from build123d import *

# Parameters (mm, degrees)
DODANIE_WYCI_GNI_CIE1_DEPTH = 6
SZKIC3_R                    = 21.25
WYTNIJ_WYCI_GNI_CIE1_DEPTH  = 10
SZKIC4_R                    = 1.55
WYTNIJ_WYCI_GNI_CIE2_DEPTH  = 10


with BuildPart() as part:
    # Szkic1 → Dodanie-wyciągnięcie1 (new body)
    with BuildSketch(Plane.XY):
        with BuildLine():
            ThreePointArc((38.780616011, 73.907751151), (41.279513808, -10.21802082), (43.778411605, 73.907751151))
            ThreePointArc((43.778411605, 73.907751151), (41.279513808, 76.48197918), (38.780616011, 73.907751151))
        make_face()
    extrude(amount=DODANIE_WYCI_GNI_CIE1_DEPTH)

    # Szkic3 → Wytnij-wyciągnięcie1 (cut)
    with BuildSketch(Plane.XY.offset(6)):
        with Locations((41.279513808, 21.88197918)):
            Circle(SZKIC3_R)
    extrude(amount=-WYTNIJ_WYCI_GNI_CIE1_DEPTH, mode=Mode.SUBTRACT)

    # Szkic4 → Wytnij-wyciągnięcie2 (cut)
    with BuildSketch(Plane.XY.offset(6)):
        with Locations((41.279513808, -5.11802082)):
            Circle(SZKIC4_R)
        with Locations((17.896827906, 35.38197918)):
            Circle(SZKIC4_R)
        with Locations((64.66219971, 35.38197918)):
            Circle(SZKIC4_R)
        with Locations((41.279513808, 66.88197918)):
            Circle(SZKIC4_R)
    extrude(amount=-WYTNIJ_WYCI_GNI_CIE2_DEPTH, mode=Mode.SUBTRACT)


solid = part.part
For this review, take the finished solid that the model builds, in its own axes (mm). Round coordinates to 2 decimals unless told otherwise and drop trailing zeros. Order: outer loops, then holes, each group sorted by start corner. A loop starts at its lowest first (then second) coordinate and runs counter-clockwise, first axis right, second up. Notation, with made-up numbers: (-17, 31.5) -> (4, 31.5) arc R13 cw to (4, 35.5) -> close; hole circle Ø10 at (49.5, 21.25). An arc over 180 degrees is marked (long way). Write item = value, one per line. Start each with the question number.
1) Insertion check: pin 1 (3 mm diameter, centred on x = 64.66, y = 35.38, fed in from -Z); pin 2 (3 mm diameter, centred on x = 36.5, z = 4.5, fed in from -Y); pin 3 (2 mm diameter, centred on y = 66, z = 4, fed in from +X); pin 4 (2 mm diameter, centred on y = 54.5, z = 1, fed in from -X). Each pin has a flat end and moves straight along its axis. Give the tip position at first contact, or say it passes through.
2) Take a section at A-A on x = 29.5. State the section outline as (y, z) points, plus the area to 3 significant figures.
3) The part is to be moulded in two halves that separate along Y. For faces 1 (the face through (40.7, 43.4, 0)), 2 (the face through (41.995, 65.507, 3.042)), 3 (the face through (51.09, 3.03, 3.04)), 4 (the face through (39.46, -10.18, 2.96)), say which applies: +Y half, -Y half, draft (parallel to the pull), parting line (faces both ways), or undercut.
4) Take a section at D-D on x = 41. State the section outline as (y, z) points, plus the area to 3 significant figures.
5) Take a section at B-B on z = 0.9. State the section outline as (x, y) points, plus the area to 3 significant figures.
6) Take a section at C-C on y = 27. State the section outline as (x, z) points.
7) To check wall thickness, follow line 1 (Y direction, x = 41.5, z = 5.5); line 2 (Y direction, x = 42, z = 2.4); line 3 (X direction, y = 3, z = 4.7). State the ranges of each line that lie inside material, in increasing order. Write a range as from..to.
Verdict:
q1.pin_1 = through
q1.pin_2 = -10.09
q1.pin_3 = 67.27
q1.pin_4 = 5.15
q2.outline = (-8.54, 0) -> (4.2, 0) -> (4.2, 6) -> (-8.54, 6) -> close; (39.57, 0) -> (72.3, 0) -> (72.3, 6) -> (39.57, 6) -> close
q2.area = 273 mm2
q3.face_1 = draft
q3.face_2 = undercut
q3.face_3 = undercut
q3.face_4 = parting line
q4.outline = (-10.22, 0) -> (-6.64, 0) -> (-6.64, 6) -> (-10.22, 6) -> close; (-3.59, 0) -> (0.63, 0) -> (0.63, 6) -> (-3.59, 6) -> close; (43.13, 0) -> (65.36, 0) -> (65.36, 6) -> (43.13, 6) -> close; (68.41, 0) -> (76.47, 0) -> (76.47, 6) -> (68.41, 6) -> close
q4.area = 229 mm2
q5.outline = (38.78, 73.91) arc R42.1 ccw (long way) to (43.78, 73.91) arc R2.5 ccw (long way) to start; hole circle Ø3.1 at (17.9, 35.38); hole circle Ø42.5 at (41.28, 21.88); hole circle Ø3.1 at (41.28, -5.12); hole circle Ø3.1 at (41.28, 66.88); hole circle Ø3.1 at (64.66, 35.38)
q5.area = 4,130 mm2
q6.outline = (-0.54, 0) -> (20.66, 0) -> (20.66, 6) -> (-0.54, 6) -> close; (61.9, 0) -> (83.1, 0) -> (83.1, 6) -> (61.9, 6) -> close
q7.line_1 = -10.22..-6.65, -3.58..0.63, 43.13..65.35, 68.42..76.47
q7.line_2 = -10.21..-6.49, -3.75..0.64, 43.12..65.51, 68.25..76.38
q7.line_3 = 10.65..31.53, 51.03..71.91
